For this review, take the finished solid that the model builds, in its own axes (mm). Face numbers are marked on the shaded views. Give positions to 0.01 mm unless a question says otherwise; leave off trailing zeros. Order: outer loops, then holes, each group sorted by start corner. A loop starts at its lowest first (then second) coordinate and runs counter-clockwise, first axis right, second up. Notation, with made-up numbers: (21.5, 66) - (76.5, 66) arc R27 cw to (76.5, 102) - close; hole circle Ø3 at (29, 2). An arc over 180 degrees is marked (long way). One line per item, written item: value.
Autodesk Inventor part; units mm, degrees
ref_plane "YZ Plane" through (0, 0, 0) normal (1, 0, 0) x (0, 1, 0)
ref_plane "XZ Plane" through (0, 0, 0) normal (0, 1, 0) x (-1, 0, 0)
ref_plane "XY Plane" through (0, 0, 0) normal (0, 0, 1) x (1, 0, 0)
sketch "Sketch1" plane through (0, 0, 0) normal (0, 0, 1) x (1, 0, 0)
  line L0 (0, 0) -> (0, 36)
  line L1 (0, 36) -> (36, 36)
  line L2 (36, 36) -> (36, 0)
  line L3 (36, 0) -> (0, 0)
  dimension "d0" = 36
  dimension "d1" = 36
extrude "Extrusion1" add sketch "Sketch1" along normal blind 57
sketch "Sketch2" plane through (0, 0, 57) normal (0, 0, 1) x (1, 0, 0)
  circle A0 centre (18, 18) radius 8
  dimension "d4" = 16
hole "Hole1" at (18, 18, 57) direction (0, 0, -1) diameter 16 depth 17
sketch "Sketch3" plane through (36, 0, 0) normal (1, 0, 0) x (0, 0, -1)
  circle A0 centre (-11, 18) radius 6
  dimension "d43" = 12
hole "Hole2" at (36, 18, 11) direction (-1, 0, 0) diameter 12 end through all
sketch "Sketch4" plane through (0, 36, 0) normal (0, 1, 0) x (1, 0, 0)
  circle A0 centre (18, -29) radius 6
  dimension "d46" = 12
hole "Hole3" at (18, 36, 29) direction (0, -1, 0) diameter 12 end through all
sketch "Sketch5" plane through (36, 0, 0) normal (1, 0, 0) x (0, 0, -1)
  circle A0 centre (-53.9561, 18) radius 3
  point P0 (0, 0)
  dimension "d41" = 6
hole "Hole4" at (36, 18, 53.9561) direction (-1, 0, 0) diameter 6 end through all
properties part number "Centerhoved" material "PC/ABS Plastic"
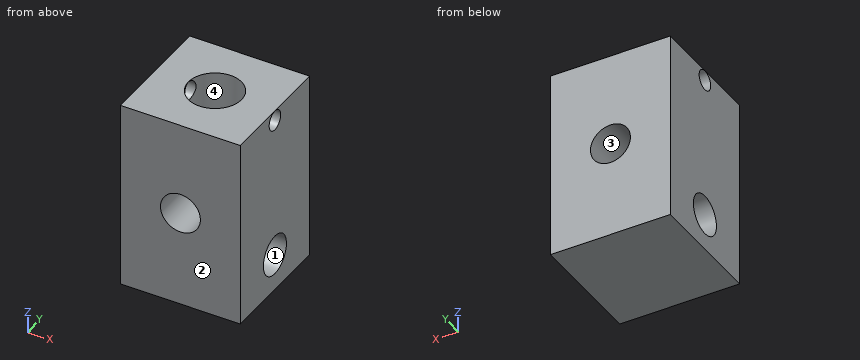
(1) Take a section at C-C (z = 29). Write out the cut boundary in (x, y).
Answers below:
outline: (0, 0) - (12, 0) - (12, 36) - (0, 36) - close; (24, 0) - (36, 0) - (36, 36) - (24, 36) - close
(2) Draft analysis for pull direction Y (two halves, no side actions). For the marked faces 1, 2, 3 and 4, state which applies: pulls with the +Y half, pulls with the -Y half, needs draft (parallel to the pull), parting line crosses it, or undercut.
Answers below:
face 1: undercut
face 2: pulls with the -Y half
face 3: needs draft
face 4: undercut
(3) Take a section at A-A (x = 18). Write out the cut boundary in (y, z), then the cut area to 3 significant figures.
Answers below:
outline: (0, 0) - (36, 0) - (36, 23) - (0, 23) - close; (0, 35) - (36, 35) - (36, 57) - (26, 57) - (26, 40) - (10, 40) - (10, 57) - (0, 57) - close; hole circle Ø12 at (18, 11)
area: 1,230 mm^2
(4) Wall thickness on line 1 (Z direction, x = 18, y = 18); line 2 (Y direction, x = 17.5, z = 52); line 3 (Z direction, x = 18, y = 13): over which ranges is each line inside the solid? List them lowest first. Write a range as from..to.
Answers below:
line 1: z = 0..5, 17..23, 35..40
line 2: y = 0..10.02, 25.98..36
line 3: z = 0..7.68, 14.32..23, 35..40
(5) Take a section at D-D (y = 31.5). Write out the cut boundary in (x, z).
Answers below:
outline: (0, 0) - (36, 0) - (36, 57) - (0, 57) - close; hole circle Ø12 at (18, 29)
(6) Take a section at B-B (y = 18). Write out the cut boundary in (x, z).
Answers below:
outline: (0, 0) - (36, 0) - (36, 5) - (0, 5) - close; (0, 17) - (36, 17) - (36, 50.96) - (26, 50.96) - (26, 40) - (10, 40) - (10, 50.96) - (0, 50.96) - close; (0, 56.96) - (10, 56.96) - (10, 57) - (0, 57) - close; (26, 56.96) - (36, 56.96) - (36, 57) - (26, 57) - close; hole circle Ø12 at (18, 29)
(7) For P1, Ø7, axis at y = 18, z = 11, coming from the -X side, flat-tipped, find the tip position at first contact; note if it passes through.
Answers below:
P1: passes through
